Work out the finished part from the listing and answer in its coordinate system (mm). A direction names the side the tool comes from. Round coordinates to 2 decimals unless told otherwise and drop trailing zeros. Write each loop counter-clockwise with the first axis right and the second up, starting at its lowest first coordinate (ties: lowest second). Pieces come first, ordered by that corner, then holes. Notation, with made-up numbers: (77.25, -23.5) - (93.25, -23.5) arc R21 cw to (93.25, -19.5) - close; hole circle Ø10 at (13, 21). An arc over 180 degrees is marked (long way). Answer as a JSON object with one key per item and string values.
```python
from build123d import *

# Parameters (mm, degrees)
SKETCH1_W           = 50.8
SKETCH1_H           = 25.4
SKETCH1_R           = 2.413
SKETCH1_R_2         = 1.143
BOSS_EXTRUDE1_DEPTH = 1.143


with BuildPart() as part:
    # Sketch1 → Boss-Extrude1 (new, symmetric)
    with BuildSketch(Plane.XY):
        Rectangle(SKETCH1_W, SKETCH1_H)
        with Locations((-12.7, 0)):
            Circle(SKETCH1_R, mode=Mode.SUBTRACT)
        with Locations((12.7, 0)):
            Circle(SKETCH1_R_2, mode=Mode.SUBTRACT)
        Polygon((7.62, 4.399409051), (0, 8.798818102), (-7.62, 4.399409051), (-7.62, -4.399409051), (0, -8.798818102), (7.62, -4.399409051), align=None, mode=Mode.SUBTRACT)
    extrude(amount=BOSS_EXTRUDE1_DEPTH, both=True)


solid = part.part
```
Item 1: A cutting plane is placed at A-A (x = 12.7). Write down the section's boundary in (y, z).
Results found:
{"outline": "(-12.7, -1.14) - (-1.14, -1.14) - (-1.14, 1.14) - (-12.7, 1.14) - close; (1.14, -1.14) - (12.7, -1.14) - (12.7, 1.14) - (1.14, 1.14) - close"}
Item 2: A cutting plane is placed at B-B (y = 0). Write down the section's boundary in (x, z), and give its area (3 significant figures).
Results found:
{"outline": "(-25.4, -1.14) - (-15.11, -1.14) - (-15.11, 1.14) - (-25.4, 1.14) - close; (-10.29, -1.14) - (-7.62, -1.14) - (-7.62, 1.14) - (-10.29, 1.14) - close; (7.62, -1.14) - (11.56, -1.14) - (11.56, 1.14) - (7.62, 1.14) - close; (13.84, -1.14) - (25.4, -1.14) - (25.4, 1.14) - (13.84, 1.14) - close", "area": "65.0 mm²"}
Item 3: For faces 5 (the flat face through (25.4, 0, 0)), 6 (the flat face through (7.62, 0, 0)), determine the directions among +Z, -Z, +X, -X, +Y, -Y from which every point of the face is accessible in a straight line to the end or side of a thin tool.
Results found:
{"face 5": "+Z, -Z, +X, +Y, -Y", "face 6": "+Z, -Z"}
Item 4: Determine the mould class of faces 1 (the flat face through (-3.76, 6.63, 0.02)), 2 (the flat face through (-25.4, 0, 0)), 3 (the flat face through (0, -12.7, 0)), 4 (the flat face through (-3.86, -6.57, 0.02)) for opening direction X: pulls with the +X half, pulls with the -X half, needs draft (parallel to the pull), parting line crosses it, or undercut.
Results found:
{"face 1": "undercut", "face 2": "pulls with the -X half", "face 3": "needs draft", "face 4": "undercut"}
Item 5: A cutting plane is placed at C-C (z = -0.1). Write down the section's boundary in (x, y).
Results found:
{"outline": "(-25.4, -12.7) - (25.4, -12.7) - (25.4, 12.7) - (-25.4, 12.7) - close; hole circle Ø4.83 at (-12.7, 0); hole (-7.62, -4.4) - (0, -8.8) - (7.62, -4.4) - (7.62, 4.4) - (0, 8.8) - (-7.62, 4.4) - close; hole circle Ø2.29 at (12.7, 0)"}
Item 6: A cutting plane is placed at D-D (x = -12.7). Write down the section's boundary in (y, z), and give its area (3 significant figures).
Results found:
{"outline": "(-12.7, -1.14) - (-2.41, -1.14) - (-2.41, 1.14) - (-12.7, 1.14) - close; (2.41, -1.14) - (12.7, -1.14) - (12.7, 1.14) - (2.41, 1.14) - close", "area": "47.0 mm²"}
Item 7: This flat-tipped pin is pushed along its axis until it touches: P1, Ø2, axis at x = 12.7, y = 0, coming from the -Z side. Where does it stop, or does it pass through?
Results found:
{"P1": "through"}
Item 8: Consider line 1 along X through (y, z) = (-1, -0.55); line 2 along Y through (x, z) = (-12.7, -0.7); line 3 along X through (y, z) = (1.75, 0.95). Determine where each line is inside the solid, lowest interval first.
Results found:
{"line 1": "-25.4 to -14.9, -10.5 to -7.62, 7.62 to 12.15, 13.25 to 25.4", "line 2": "-12.7 to -2.41, 2.41 to 12.7", "line 3": "-25.4 to -14.36, -11.04 to -7.62, 7.62 to 25.4"}
